from build123d import *

# Parameters (mm, degrees)
EXTRUDE_THIN1_DEPTH = 25.4
FILLET1_R           = 3.175
SKETCH2_R           = 3.175
EXTRUDE1_DEPTH      = 25.4


with BuildPart() as part:
    # Sketch1 → Extrude-Thin1 (new body)
    with BuildSketch(Plane.XY):
        with BuildLine():
            Line((0, 25.4), (0, 4.7625))
            ThreePointArc((0, 4.7625), (1.394903955, 1.394903955), (4.7625, 0))
            Line((4.7625, 0), (71.4375, 0))
            ThreePointArc((71.4375, 0), (74.805096045, 1.394903955), (76.2, 4.7625))
            Line((76.2, 4.7625), (76.2, 25.4))
            Line((76.2, 25.4), (73.025, 25.4))
            Line((73.025, 25.4), (73.025, 4.7625))
            ThreePointArc((73.025, 4.7625), (72.560032015, 3.639967985), (71.4375, 3.175))
            Line((71.4375, 3.175), (4.7625, 3.175))
            ThreePointArc((4.7625, 3.175), (3.639967985, 3.639967985), (3.175, 4.7625))
            Line((3.175, 4.7625), (3.175, 25.4))
            Line((3.175, 25.4), (0, 25.4))
        make_face()
    extrude(amount=-EXTRUDE_THIN1_DEPTH)

    # Fillet1
    fillet1_edges = [part.edges().sort_by_distance(p)[0] for p in [
        (1.5875, 25.4, 0),
        (74.6125, 25.4, 0),
        (1.5875, 25.4, -25.4),
        (74.6125, 25.4, -25.4),
    ]]
    fillet(fillet1_edges, radius=FILLET1_R)

    # Sketch2 → Extrude1 (cut)
    with BuildSketch(Plane(origin=(0, 3.175, 0), x_dir=(-1, 0, 0), z_dir=(0, 1, 0))):
        with Locations(Location((-21.43125, -12.7, 0), (0, 0, 90))):
            Circle(SKETCH2_R)
        with Locations(Location((-54.76875, -12.7, 0), (0, 0, 270))):
            Circle(SKETCH2_R)
    extrude(amount=-EXTRUDE1_DEPTH, mode=Mode.SUBTRACT)


solid = part.part
Part model, mm, in its own coordinate system. A direction names the side the tool comes from. Round coordinates to 2 decimals unless told otherwise and drop trailing zeros. Loops run counter-clockwise (first coordinate to the right, second up) from the corner with the lowest first, then second, coordinate; pieces in that order, holes last. Notation, with made-up numbers: (-34, -29) - (16, -29) arc R17 ccw to (16, -20) - close; hole circle Ø1 at (5.5, -5). An arc over 180 degrees is marked (long way). Answer as a JSON object with one key per item and string values.
Item 1: Band-saw the part on A-A on z = -12.7. List the corners of the cut face in (x, y) (1 decimal).
Output:
{"outline": "(0, 4.8) arc R4.8 ccw to (4.8, 0) - (18.3, 0) - (18.3, 3.2) - (4.8, 3.2) arc R1.6 cw to (3.2, 4.8) - (3.2, 25.4) - (0, 25.4) - close; (24.6, 0) - (51.6, 0) - (51.6, 3.2) - (24.6, 3.2) - close; (57.9, 0) - (71.4, 0) arc R4.8 ccw to (76.2, 4.8) - (76.2, 25.4) - (73, 25.4) - (73, 4.8) arc R1.6 cw to (71.4, 3.2) - (57.9, 3.2) - close"}
Item 2: Band-saw the part on C-C on x = 57. List the corners of the cut face in (y, z) (3 decimals), plus the area to 3 significant figures.
Output:
{"outline": "(0, -25.4) - (3.175, -25.4) - (3.175, -14.959) - (0, -14.959) - close; (0, -10.441) - (3.175, -10.441) - (3.175, 0) - (0, 0) - close", "area": "66.3 mm2"}
Item 3: Band-saw the part on B-B on y = 8.75. List the corners of the cut face in (x, z) (3 decimals).
Output:
{"outline": "(0, -25.4) - (3.175, -25.4) - (3.175, 0) - (0, 0) - close; (73.025, -25.4) - (76.2, -25.4) - (76.2, 0) - (73.025, 0) - close"}
Item 4: Tool access for faces 1 (the face through (72.57, 3.65, -12.52)), 2 (the face through (38, 0, -13)): list every direction of +Z, -Z, +X, -X, +Y, -Y with a clear straight run to the whole face (end or side of a thin tool).
Output:
{"face 1": "+Z, -Z, +Y", "face 2": "+Z, -Z, +X, -X, -Y"}
Item 5: Pull direction X, two halves, no side cores. Call faces 3 (the face through (1.57, 24.49, -0.95)), 4 (the face through (3.175, 15, -13)), 5 (the face through (74.77, 1.36, -12.52)): pulls with the +X half, pulls with the -X half, needs draft (parallel to the pull), parting line crosses it, or undercut.
Output:
{"face 3": "needs draft", "face 4": "undercut", "face 5": "pulls with the +X half"}
Item 6: Wall check: L1, parallel to X at y = 15.75, z = -12.75 (3 decimals); L2, parallel to X at y = 2.05, z = -12.7; L3, parallel to X at y = 0.85, z = -12.7. Give the ranges that are in metal, low to high.
Output:
{"L1": "0 to 3.175, 73.025 to 76.2", "L2": "0.85 to 18.26, 24.61 to 51.59, 57.94 to 75.35", "L3": "2.05 to 18.26, 24.61 to 51.59, 57.94 to 74.15"}
Item 7: Pin check, flat tip, straight feed: pin 1 (4 mm diameter, centred on x = 52.5, z = -8, fed in from +Y) (3 decimals). Stop position of the tip, or through.
Output:
{"pin 1": "y = 3.175"}
Item 8: Band-saw the part on D-D on z = -7.5. List the corners of the cut face in (x, y) (1 decimal).
Output:
{"outline": "(0, 4.8) arc R4.8 ccw to (4.8, 0) - (71.4, 0) arc R4.8 ccw to (76.2, 4.8) - (76.2, 25.4) - (73, 25.4) - (73, 4.8) arc R1.6 cw to (71.4, 3.2) - (4.8, 3.2) arc R1.6 cw to (3.2, 4.8) - (3.2, 25.4) - (0, 25.4) - close"}
